```python
from build123d import *

# Parameters (mm, degrees)
SKETCH_1_R          = 31
SKETCH_1_R_2        = 22.5
SKETCH_1_R_3        = 10.5
EXTRUDE_1_DEPTH     = 72
EXTRUDE_START       = 8
SKETCH_1_3_R        = 22.5
SKETCH_1_3_R_2      = 10.5
EXTRUDE_2_DEPTH     = 8
SKETCH_2_R          = 2.5
SKETCH_2_R_2        = 2
CUT_EXTRUDE_3_DEPTH = 7


with BuildPart() as part:
    # Sketch 1 → Extrude 1 (new body)
    # profile 1 of 2: a face of its own
    with BuildSketch(Plane.XY):
        Circle(SKETCH_1_R)
        Circle(SKETCH_1_R_2, mode=Mode.SUBTRACT)
    # profile 2 of 2: a face of its own
    with BuildSketch(Plane.XY):
        Circle(SKETCH_1_R_2)
        Circle(SKETCH_1_R_3, mode=Mode.SUBTRACT)
    extrude(amount=-EXTRUDE_1_DEPTH)

    # Sketch 1_3 → Extrude 2 (add)
    with BuildSketch(Plane.XY.offset(EXTRUDE_START)):
        Circle(SKETCH_1_3_R)
        Circle(SKETCH_1_3_R_2, mode=Mode.SUBTRACT)
    extrude(amount=-EXTRUDE_2_DEPTH)

    # Sketch 2 → Cut-Extrude 3 (cut)
    with BuildSketch(Plane.XY):
        with Locations((0, 26.75)):
            Circle(SKETCH_2_R)
        with Locations((18.915106397, 18.915106397)):
            Circle(SKETCH_2_R_2)
        with Locations(Location((0, -26.75, 0), (0, 0, 180))):
            Circle(SKETCH_2_R)
        with Locations((18.915106397, -18.915106397)):
            Circle(SKETCH_2_R_2)
        with Locations((-18.915106397, -18.915106397)):
            Circle(SKETCH_2_R_2)
        with Locations((-18.915106397, 18.915106397)):
            Circle(SKETCH_2_R_2)
    extrude(amount=-CUT_EXTRUDE_3_DEPTH, mode=Mode.SUBTRACT)


solid = part.part
```
Build history of the part. All positions in model axes, mm. A direction names the side the tool comes from. Coordinates: 2 decimals unless noted, no trailing zeros. Order: outer loops, then holes, each group sorted by start corner. A loop starts at its lowest first (then second) coordinate and runs counter-clockwise, first axis right, second up.
Item 1: Drop flat-ended pins along their axis: pin 1 Ø3 at (x, y) = (0, 26.75) entering from +Z; pin 2 Ø4 at (x, y) = (-1, 28) entering from +Z; pin 3 Ø6 at (y, z) = (-10, -61.5) entering from -X. Give the stop position or say it passes through.
Filled in:
pin 1: stops at z = -7
pin 2: stops at z = 0
pin 3: stops at x = -30.2
Item 2: Mould opens along Y. For faces 1 (the cylindrical face through (-4.036, 30.736, -35.496)), 2 (the cylindrical face through (0.33, -29.23, -3.45)), 3 (the flat face through (0, -13, -72)), 4 (the cylindrical face through (-20.502, 17.698, -3.451)) say: released by +Y, released by -Y, zero draft, split by the parting line, or undercut.
Filled in:
face 1: split by the parting line
face 2: undercut
face 3: zero draft
face 4: undercut
Item 3: Saw through at C-C on z = -19.5. List the corners of the cut face in (x, y), then the cut area to 3 significant figures.
Filled in:
outline: circle Ø62 at (0, 0); hole circle Ø21 at (0, 0)
area: 2,670 mm2
Item 4: Saw through at D-D on y = 26.75. List the corners of the cut face in (x, z), then the cut area to 3 significant figures.
Filled in:
outline: (-15.67, -72) - (15.67, -72) - (15.67, 0) - (2.5, 0) - (2.5, -7) - (-2.5, -7) - (-2.5, 0) - (-15.67, 0) - close
area: 2,220 mm2
Item 5: Saw through at A-A on y = 0. List the corners of the cut face in (x, z), then the cut area to 3 significant figures.
Filled in:
outline: (-31, -72) - (-10.5, -72) - (-10.5, 8) - (-22.5, 8) - (-22.5, 0) - (-31, 0) - close; (10.5, -72) - (31, -72) - (31, 0) - (22.5, 0) - (22.5, 8) - (10.5, 8) - close
area: 3,140 mm2
Item 6: Tool access for faces 5 (the cylindrical face through (10, 3.2, -31.4)), 6 (the cylindrical face through (-0.33, 29.23, -3.45)): list every direction of +Z, -Z, +X, -X, +Y, -Y with a clear straight run to the whole face (end or side of a thin tool).
Filled in:
face 5: +Z, -Z
face 6: +Z
Item 7: Drill centre lines: L1, parallel to Y at x = 0, z = -5; L2, parallel to Z at x = -6.5, y = -23.5; L3, parallel to Y at x = -6, z = -38. Where is each one in solid material? Low to high.
Filled in:
L1: y = -31 to -29.25, -24.25 to -10.5, 10.5 to 24.25, 29.25 to 31
L2: z = -72 to 0
L3: y = -30.41 to -8.62, 8.62 to 30.41
Item 8: Saw through at B-B on x = 0. List the corners of the cut face in (y, z).
Filled in:
outline: (-31, -72) - (-10.5, -72) - (-10.5, 8) - (-22.5, 8) - (-22.5, 0) - (-24.25, 0) - (-24.25, -7) - (-29.25, -7) - (-29.25, 0) - (-31, 0) - close; (10.5, -72) - (31, -72) - (31, 0) - (29.25, 0) - (29.25, -7) - (24.25, -7) - (24.25, 0) - (22.5, 0) - (22.5, 8) - (10.5, 8) - close
